```python
from build123d import *

# Parameters (mm, degrees)
F0_W     = 42
F0_H     = 42
F1_DEPTH = 39.5
F2_R     = 1.5
F3_DEPTH = 10
F2_R_2   = 11
F4_DEPTH = 2
F5_R     = 2.5
F6_DEPTH = 21
F8_DEPTH = 15
F9_SIZE  = 3


with BuildPart() as f1:
    # F0 (on Top) → F1 (new body)
    with BuildSketch(Plane.XY):
        Rectangle(F0_W, F0_H)
    extrude(amount=F1_DEPTH)

    # F2 (on face) → F3 (cut)
    with BuildSketch(Plane.XY.offset(39.5)):
        with Locations((-15.5, -15.5)):
            Circle(F2_R)
        with Locations((-15.5, 15.5)):
            Circle(F2_R)
        with Locations((15.5, 15.5)):
            Circle(F2_R)
        with Locations((15.5, -15.5)):
            Circle(F2_R)
    extrude(amount=-F3_DEPTH, mode=Mode.SUBTRACT)

    # F2 (on face) → F4 (join)
    with BuildSketch(Plane.XY.offset(39.5)):
        Circle(F2_R_2)
    extrude(amount=F4_DEPTH)

    # F5 (on face) → F6 (join)
    with BuildSketch(Plane.XY.offset(41.5)):
        Circle(F5_R)
    extrude(amount=F6_DEPTH)

    # F7 (on face) → F8 (cut)
    with BuildSketch(Plane.XY.offset(62.5)):
        with BuildLine():
            ThreePointArc((1.5, 2), (0, 2.5), (-1.5, 2))
            Line((-1.5, 2), (1.5, 2))
        make_face()
    extrude(amount=-F8_DEPTH, mode=Mode.SUBTRACT)

    # F9
    f9_edges = [f1.edges().sort_by_distance(p)[0] for p in [
        (21, -21, 19.75),
        (21, 21, 19.75),
        (-21, -21, 19.75),
        (-21, 21, 19.75),
    ]]
    chamfer(f9_edges, length=F9_SIZE)


solid = f1.part
```
The listing builds one solid part. Answer for the finished solid, in the listing's coordinates (mm). A direction names the side the tool comes from. Coordinates: 2 decimals unless noted, no trailing zeros. Write each loop counter-clockwise with the first axis right and the second up, starting at its lowest first coordinate (ties: lowest second). Pieces come first, ordered by that corner, then holes. Notation, with made-up numbers: M 84.5,18 L 117.5,18 A17 cw 117.5,38 Z; hole C -10,22 d1. An arc over 180 degrees is marked long. Use a Markdown table: item, result. Add a question column.
1. Section A-A (x = 15.5) is taken. Give the vertices of the cut face in (y, z).
2. Given P1, Ø1.5, axis at x = -15, y = -15, coming from the +Z side; P2, Ø5, axis at x = -15.5, y = -15.5, coming from the +Z side; P3, Ø0.5, axis at x = -0.5, y = 2.5, coming from the +Z side, each flat-ended and moving along its own axis, determine where each tip first touches the part or whether it passes through.
3. Section C-C (x = 0) is taken. Give the vertices of the cut face in (y, z), plus the area to 3 significant figures.
4. Section D-D (y = 10) is taken. Give the vertices of the cut face in (x, z), plus the area to 3 significant figures.
5. For a pull along Y with two mould halves and no side action, classify faces 1 (the flat face through (-19, -20, 19)), 2 (the flat face through (-16, -15, 29.5)), 3 (the flat face through (0, 0, 62.5)) as +Y half, -Y half, draft (parallel to the pull), parting line (faces both ways), or undercut.
6. Straight lines are drawn through the part: line 1 along Y through (x, z) = (-15.5, 36.25); line 2 along X through (y, z) = (15, 37); line 3 along Z through (x, y) = (19, -8). For each, find the intervals that lie inside material, in ascending order. Write a range as [from, to].
7. Which of the six approach directions +Z, -Z, +X, -X, +Y, -Y give full straight-line access (tool end or side, diameter ignored) to faces 4 (the cylindrical face through (14, 15.57, 34.57)), 5 (the flat face through (-21, 0, 19))?
8. Section B-B (y = 0) is taken. Give the vertices of the cut face in (x, z).
Data:
| question | item | result |
|---|---|---|
| 1 | outline | M -21,0 L 21,0 L 21,39.5 L 17,39.5 L 17,29.5 L 14,29.5 L 14,39.5 L -14,39.5 L -14,29.5 L -17,29.5 L -17,39.5 L -21,39.5 Z |
| 2 | P1 | stops at z = 29.5 |
| 2 | P2 | stops at z = 39.5 |
| 2 | P3 | stops at z = 47.5 |
| 3 | outline | M -21,0 L 21,0 L 21,39.5 L 11,39.5 L 11,41.5 L 2.5,41.5 L 2.5,47.5 L 2,47.5 L 2,62.5 L -2.5,62.5 L -2.5,41.5 L -11,41.5 L -11,39.5 L -21,39.5 Z |
| 3 | area | 1,800 mm2 |
| 4 | outline | M -21,0 L 21,0 L 21,39.5 L 4.58,39.5 L 4.58,41.5 L -4.58,41.5 L -4.58,39.5 L -21,39.5 Z |
| 4 | area | 1,680 mm2 |
| 5 | face 1 | -Y half |
| 5 | face 2 | undercut |
| 5 | face 3 | draft |
| 6 | line 1 | y = [-21, -17], [-14, 14], [17, 21] |
| 6 | line 2 | x = [-21, -16.91], [-14.09, 14.09], [16.91, 21] |
| 6 | line 3 | z = [0, 39.5] |
| 7 | face 4 | +Z |
| 7 | face 5 | +Z, -Z, -X, +Y, -Y |
| 8 | outline | M -21,0 L 21,0 L 21,39.5 L 11,39.5 L 11,41.5 L 2.5,41.5 L 2.5,62.5 L -2.5,62.5 L -2.5,41.5 L -11,41.5 L -11,39.5 L -21,39.5 Z |
